```python
from build123d import *

# Parameters (mm, degrees)
F0_W        = 147.209584713
F0_H        = 117.8593859076
F1_DEPTH    = 126
F2_R        = 5
F3_T        = -2.5
F4_T1_DEPTH = 133.5
F4_S5_W     = 5
F4_S5_H     = 5
F4_T6_DEPTH = 5


# Not quite as in the source:
# - a fillet or chamfer that OpenCascade refuses, or shapes differently, is made with other operations: its cross-section is extruded or revolved along the edge and cut away or added


with BuildPart() as f1:
    # F0 (on Top) → F1 (new body)
    with BuildSketch(Plane.XY):
        Rectangle(F0_W, F0_H)
    extrude(amount=F1_DEPTH)

    # F2
    f2_edges = [f1.edges().sort_by_distance(p)[0] for p in [
        (-73.604792, -58.929693, 63),
        (73.604792, -58.929693, 63),
        (0, -58.929693, 126),
        (-73.604792, 0, 126),
        (0, 58.929693, 126),
        (73.604792, 0, 126),
        (-73.604792, 58.929693, 63),
    ]]
    fillet(f2_edges, radius=F2_R)

    # F3
    f3_openings = [f1.faces().sort_by_distance(p)[0] for p in [
        (0.022436, 0.017894, 0),
    ]]
    offset(amount=F3_T, openings=f3_openings)

    # F4: fillet of radius 5 on 1 edges, made by hand

    # F4_s2 → F4_t1 (cut)
    with BuildSketch(Plane.XY.offset(-12.5)):
        with BuildLine():
            ThreePointArc((73.6047923565, 53.9296929538), (72.1403262624, 57.4652268598), (68.6047923565, 58.9296929538))
            Line((68.6047923565, 58.9296929538), (73.6047923565, 58.9296929538))
            Line((73.6047923565, 58.9296929538), (73.6047923565, 53.9296929538))
        make_face()
    extrude(amount=F4_T1_DEPTH, mode=Mode.SUBTRACT)


with BuildPart() as f4_tool4:
    # F4_s5 → F4_t6 (new body)
    with BuildSketch(Plane.YZ.offset(68.6047923565)):
        with Locations((56.4296929538, 123.5)):
            Rectangle(F4_S5_W, F4_S5_H)
    extrude(amount=F4_T6_DEPTH)

    # F4_s7 → F4_t8 (revolve, cut)
    with BuildSketch(Plane(origin=(68.6047923565, 53.9296929538, 121), x_dir=(0, -0.7071067812, -0.7071067812), z_dir=(0, -0.7071067812, 0.7071067812))):
        with BuildLine():
            ThreePointArc((0, -5), (5, 0), (0, 5))
            Line((0, 5), (0, -5))
        make_face()
    revolve(axis=Axis((68.6047923565, 53.9296929538, 121), (1, 0, 0)), mode=Mode.SUBTRACT)


with BuildPart() as f1_1:
    add(f1.part)

    # F4_t3: cut F4_tool4
    add(f4_tool4.part, mode=Mode.SUBTRACT)


solid = f1_1.part
```
Read the model definition and answer for the solid it produces. Units are mm, in the model's axes. A direction names the side the tool comes from. Coordinates: 2 decimals unless noted, no trailing zeros. Order: outer loops, then holes, each group sorted by start corner. A loop starts at its lowest first (then second) coordinate and runs counter-clockwise, first axis right, second up. Notation, with made-up numbers: (-26, 5) - (27, 5) arc R19 ccw to (27, 14) - close; hole circle Ø10 at (89.25, 67). An arc over 180 degrees is marked (long way). Answer as a JSON object with one key per item and string values. Group by question number.
Item 1: A flat-ended cylindrical pin translates along its axis: P1, Ø5, axis at x = -50.5, y = 12.5, coming from the -Z side. Find the tip coordinate at first contact, or state that the pin passes through.
Item 2: Section C-C (x = 13) is taken. Give the vertices of the cut face in (y, z), plus the area to 3 significant figures.
Item 3: The mould has two halves that part along Y. Classify faces 3 (the face through (-1, -58.93, 60)), 4 (the face through (-72.179, 57.426, 61.347)), 5 (the face through (-71.105, -1, 60)), 6 (the face through (72.179, 0.755, 124.496)): +Y half, -Y half, draft (parallel to the pull), parting line (faces both ways), or undercut.
Item 4: Section A-A (y = 1) is taken. Give the vertices of the cut face in (x, z).
Item 5: Section B-B (z = 35) is taken. Give the vertices of the cut face in (x, y).
Item 6: A tool of negligible diameter and unlimited length cuts with its end or side. For faces 1 (the face through (71.105, 0, 60)), 2 (the face through (1, 57.5, 124.5)), from which of +Z, -Z, +X, -X, +Y, -Y can it reach the whole face along a straight path? Write none if from no direction.
Item 7: Consider probe 1 along Y at (x, z) = (-53.5, 86.5); probe 2 along X at (y, z) = (14.5, 19.5); probe 3 along Z at (x, y) = (-25, -13.5). Determine where each line is inside the solid, lowest interval first. Write a range as from..to.
Results are:
{
 "1": {"P1": "stops at z = 123.5"},
 "2": {"outline": "(-58.93, 0) - (-56.43, 0) - (-56.43, 121) arc R2.5 cw to (-53.93, 123.5) - (53.93, 123.5) arc R2.5 cw to (56.43, 121) - (56.43, 0) - (58.93, 0) - (58.93, 121) arc R5 ccw to (53.93, 126) - (-53.93, 126) arc R5 ccw to (-58.93, 121) - close", "area": "904 mm^2"},
 "3": {"face 3": "-Y half", "face 4": "+Y half", "face 5": "undercut", "face 6": "draft"},
 "4": {"outline": "(-73.6, 0) - (-71.1, 0) - (-71.1, 121) arc R2.5 cw to (-68.6, 123.5) - (68.6, 123.5) arc R2.5 cw to (71.1, 121) - (71.1, 0) - (73.6, 0) - (73.6, 121) arc R5 ccw to (68.6, 126) - (-68.6, 126) arc R5 ccw to (-73.6, 121) - close"},
 "5": {"outline": "(-73.6, -53.93) arc R5 ccw to (-68.6, -58.93) - (68.6, -58.93) arc R5 ccw to (73.6, -53.93) - (73.6, 53.93) arc R5 ccw to (68.6, 58.93) - (-68.6, 58.93) arc R5 ccw to (-73.6, 53.93) - close; hole (-71.1, -53.93) arc R2.5 ccw to (-68.6, -56.43) - (68.6, -56.43) arc R2.5 ccw to (71.1, -53.93) - (71.1, 56.43) - (-68.6, 56.43) arc R2.5 ccw to (-71.1, 53.93) - close"},
 "6": {"face 1": "-Z", "face 2": "+Z, +X, -X, +Y"},
 "7": {"probe 1": "y = -58.93..-56.43, 56.43..58.93", "probe 2": "x = -73.6..-71.1, 71.1..73.6", "probe 3": "z = 123.5..126"}
}
